from build123d import *

# Parameters (mm, degrees)
CROQUIS1_W                 = 4
CROQUIS1_H                 = 13
CHAFL_N1_SIZE              = 0.2
CORTAR_EXTRUIR1_DEPTH      = 9.61684397
CORTAR_EXTRUIR1_DEPTH_BACK = 9.61684397
CROQUIS2_R                 = 2.15


with BuildPart() as part:
    # Croquis1 → Revolución1 (revolve)
    with BuildSketch(Plane(origin=(0, 0, 0), x_dir=(1, 0, 0), z_dir=(0, 1, 0)), mode=Mode.PRIVATE) as revoluci_n1_sk:
        with Locations((2, 0)):
            Rectangle(CROQUIS1_W, CROQUIS1_H)
    revolve(revoluci_n1_sk.sketch.rotate(Axis((0, 0, -6.5), (0, 0, 1)), 180), axis=Axis((0, 0, -6.5), (0, 0, 1)))

    # Chaflán1
    chafl_n1_edges = [part.edges().sort_by_distance(p)[0] for p in [
        (4, 0, 6.5),
        (4, 0, -6.5),
    ]]
    chamfer(chafl_n1_edges, length=CHAFL_N1_SIZE)

    # Croquis2 → Cortar-Extruir1 (cut, two sides: drawn at the far end of the back side and taken through both)
    with BuildSketch(Plane(origin=(0, 0, 0), x_dir=(1, 0, 0), z_dir=(0, 1, 0)).offset(-CORTAR_EXTRUIR1_DEPTH_BACK)):
        with Locations(Location((0, 0, 0), (0, 0, 270))):
            Circle(CROQUIS2_R)
    extrude(amount=CORTAR_EXTRUIR1_DEPTH + CORTAR_EXTRUIR1_DEPTH_BACK, mode=Mode.SUBTRACT)

    # Croquis3 → Cortar-Revolución1 (revolve, cut)
    with BuildSketch(Plane(origin=(0, 0, 0), x_dir=(0, 0, -1), z_dir=(1, 0, 0))):
        Polygon((0, 2.827658977), (-1.417641815, 2.827658977), (-3.618319017, 4.807613665), (0, 4.807613665), align=None)
    cortar_revoluci_n1 = revolve(axis=Axis((0, 0, 0), (0, 1, 0)), mode=Mode.SUBTRACT)

    # Simetría1: Cortar-Revolución1 across plane
    add(cortar_revoluci_n1.mirror(Plane.ZX), mode=Mode.SUBTRACT)


solid = part.part
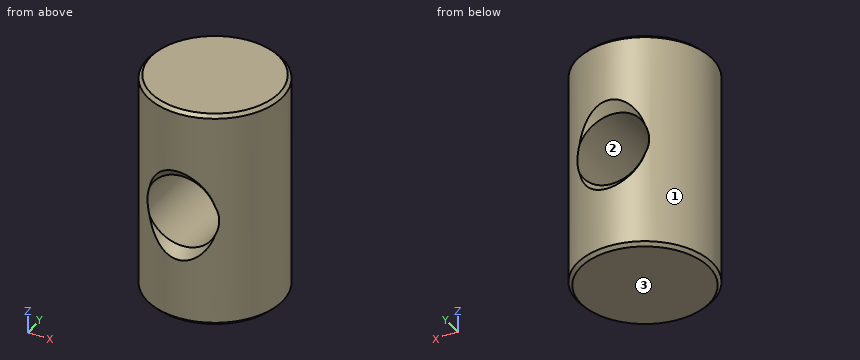
The listing builds one solid part. Answer for the finished solid, in the listing's coordinates (mm). Face numbers are marked on the shaded views. Give positions to 0.01 mm unless a question says otherwise; leave off trailing zeros. Order: outer loops, then holes, each group sorted by start corner. A loop starts at its lowest first (then second) coordinate and runs counter-clockwise, first axis right, second up. Notation, with made-up numbers: (6, -21) - (25, -21) arc R35 ccw to (25, 14) - close; hole circle Ø11 at (-26.5, 73.25). An arc over 180 degrees is marked (long way). Use one line per item in the form item = value.
1) The mould has two halves that part along X. Classify the marked faces 1, 2 and 3: released by +X, released by -X, zero draft, split by the parting line, or undercut.
Verdict:
face_1 = split by the parting line
face_2 = undercut
face_3 = zero draft
2) Find section A-A on y = 0. Determine the outline of the cut face in (x, z), and give its area (3 significant figures).
Verdict:
outline = (-4, -6.3) - (-3.8, -6.5) - (3.8, -6.5) - (4, -6.3) - (4, 6.3) - (3.8, 6.5) - (-3.8, 6.5) - (-4, 6.3) - close; hole circle Ø4.3 at (0, 0)
area = 89.4 mm^2
3) Consider probe 1 along Z at (x, y) = (0, 0.25); probe 2 along X at (y, z) = (-1.25, 0); probe 3 along X at (y, z) = (-1.25, -2.5). Determine where each line is inside the solid, lowest interval first. Write a range as [from, to].
Verdict:
probe_1 = [-6.5, -2.15], [2.15, 6.5]
probe_2 = [-3.8, -2.15], [2.15, 3.8]
probe_3 = [-3.8, 3.8]
4) Find section B-B on z = 5.5. Determine the outline of the cut face in (x, y), and give its area (3 significant figures).
Verdict:
outline = circle Ø8 at (0, 0)
area = 50.3 mm^2
5) Find section C-C on z = 0. Determine the outline of the cut face in (x, y).
Verdict:
outline = (-2.15, -3.37) - (-2.15, 3.37) arc R4 ccw to start; (2.15, -3.37) arc R4 ccw to (2.15, 3.37) - close
6) Each of these flat-tipped pins is pushed along its axis until it touches: pin 1 (2 mm diameter, centred on x = -1.5, z = 3.5, fed in from -Y); pin 2 (2 mm diameter, centred on y = -2.5, z = 4.5, fed in from -X). Where does it stop, or does it pass through?
Verdict:
pin_1 = -3.97
pin_2 = -3.71
